Autodesk Inventor part; units mm, degrees
ref_plane "YZ Plane" through (0, 0, 0) normal (1, 0, 0) x (0, 1, 0)
ref_plane "XZ Plane" through (0, 0, 0) normal (0, 1, 0) x (-1, 0, 0)
ref_plane "XY Plane" through (0, 0, 0) normal (0, 0, 1) x (1, 0, 0)
sketch "Sketch1" plane through (0, 0, 0) normal (0, 1, 0) x (-1, 0, 0)
  line L0 (63.6448, -68.929) -> (37.6448, -68.929)
  line L1 (37.6448, -68.929) -> (37.6448, -42.929)
  line L2 (37.6448, -42.929) -> (63.6448, -42.929)
  line L3 (63.6448, -42.929) -> (63.6448, -68.929)
  point P0 (0, 0)
  dimension "d0" = 26
  dimension "d1" = 26
extrude "Extrusion1" add sketch "Sketch1" along normal blind 1.2
sketch "Sketch2" plane through (0, 1.2, 0) normal (0, 1, 0) x (1, 0, 0)
  line L0 (-63.6448, 68.929) -> (-63.6448, 42.929)
  line L1 (-37.6448, 42.929) -> (-37.6448, 68.929)
  line L2 (-63.6448, 64.229) -> (-37.6448, 64.229)
  line L3 (-37.6448, 64.229) -> (-37.6448, 47.629)
  line L4 (-37.6448, 47.629) -> (-63.6448, 47.629)
  line L5 (-63.6448, 47.629) -> (-63.6448, 64.229)
  line L6 (-37.6448, 68.929) -> (-63.6448, 68.929)
  point P0 (0, 0)
  point P1 (-63.6448, 47.629)
  dimension "d4" = 4.7
  dimension "d5" = 16.6
extrude "Extrusion2" add sketch "Sketch2" along normal blind 2 contours L2 L1 L4 L0
sketch "Sketch3" plane through (0, 1.2, 0) normal (0, 1, 0) x (1, 0, 0)
  circle A0 centre (-61.6448, 66.929) radius 1
  circle A1 centre (-39.6448, 66.929) radius 1
  circle A2 centre (-39.6448, 44.929) radius 1
  circle A3 centre (-61.8448, 44.929) radius 1
  line L0 (-63.6448, 68.929) -> (-63.6448, 64.229)
  line L1 (-37.6448, 68.929) -> (-63.6448, 68.929)
  line L2 (-37.6448, 64.229) -> (-37.6448, 68.929)
  line L3 (-37.6448, 42.929) -> (-37.6448, 47.629)
  line L4 (-63.6448, 42.929) -> (-37.6448, 42.929)
  line L5 (-63.6448, 47.629) -> (-63.6448, 42.929)
  point P0 (0, 0)
  point P1 (-63.6448, 45.279)
  dimension "d8" = 2
  dimension "d9" = 2
  dimension "d10" = 2
  dimension "d11" = 2
  dimension "d12" = 2
  dimension "d13" = 2
  dimension "d14" = 2
  dimension "d15" = 2
  dimension "d16" = 2
  dimension "d17" = 2
  dimension "d18" = 2
  dimension "d19" = 1.8
extrude "Extrusion3" cut sketch "Sketch3" against normal through all
sketch "Sketch4" plane through (0, 0, 0) normal (0, -1, 0) x (1, 0, 0)
  line L0 (-45.8948, -68.929) -> (-55.8948, -68.929)
  line L1 (-55.8948, -68.929) -> (-55.8948, -66.429)
  line L2 (-55.8948, -66.429) -> (-45.8948, -66.429)
  line L3 (-45.8948, -66.429) -> (-45.8948, -68.929)
  line L4 (-37.6448, -68.929) -> (-63.6448, -68.929)
  line L5 (-37.6448, -42.929) -> (-37.6448, -68.929)
  point P0 (0, 0)
  dimension "d22" = 10
  dimension "d23" = 2.5
  dimension "d24" = 0
  dimension "d25" = 8.25
extrude "Extrusion4" add sketch "Sketch4" along normal blind 2.5
sketch "Sketch5" plane through (0, -2.5, 0) normal (0, -1, 0) x (1, 0, 0)
  line L0 (-64.9448, -68.229) -> (-76.9448, -68.229)
  line L1 (-76.9448, -68.229) -> (-76.9448, -56.229)
  line L2 (-76.9448, -56.229) -> (-64.9448, -56.229)
  line L3 (-64.9448, -56.229) -> (-64.9448, -68.229)
  line L4 (-64.9448, -55.629) -> (-76.9448, -55.629)
  line L5 (-76.9448, -55.629) -> (-76.9448, -43.629)
  line L6 (-76.9448, -43.629) -> (-64.9448, -43.629)
  line L7 (-64.9448, -43.629) -> (-64.9448, -55.629)
  line L8 (-55.8948, -68.929) -> (-63.6448, -68.929)
  line L9 (-63.6448, -68.929) -> (-63.6448, -42.929)
  line L10 (-63.6448, -42.929) -> (-37.6448, -42.929)
  point P0 (0, 0)
  dimension "d28" = 12
  dimension "d29" = 12
  dimension "d30" = 12
  dimension "d31" = 12
  dimension "d32" = 0.7
  dimension "d33" = 1.3
  dimension "d34" = 0.7
extrude "Extrusion5" add sketch "Sketch5" against normal blind 3.7
sketch "Sketch7" plane through (0, 1.2, 0) normal (0, 1, 0) x (1, 0, 0)
  circle A0 centre (-70.9448, 62.229) radius 3.25
  circle A1 centre (-70.9448, 49.629) radius 3.25
  line L0 (-64.9448, 68.229) -> (-76.9448, 68.229)
  line L1 (-76.9448, 68.229) -> (-76.9448, 43.629)
  line L2 (-64.9448, 55.629) -> (-76.9448, 55.629)
  line L3 (-76.9448, 55.629) -> (-76.9448, 43.629)
  point P0 (0, 0)
  point P1 (-76.9448, 56.229)
  dimension "d47" = 6.5
  dimension "d48" = 6.5
  dimension "d49" = 6
  dimension "d50" = 6
  dimension "d51" = 6
  dimension "d52" = 6
extrude "Extrusion7" add sketch "Sketch7" along normal blind 8.8
draft "FaceDraft3" angle 2.5 pull direction (0, 1, 0) faces at (-67.7053, 7.0667, -61.9675) fixed edges at (-74.1948, 1.2, -62.229)
draft "FaceDraft4" angle 2.5 pull direction (0, 1, 0) faces at (-67.7053, 7.0667, -49.3675) fixed edges at (-74.1948, 1.2, -49.629)
sketch "Sketch8" plane through (0, -2.5, 0) normal (0, -1, 0) x (1, 0, 0)
  line L0 (-78.2948, -34.929) -> (-36.2948, -34.929)
  line L1 (-36.2948, -34.929) -> (-36.2948, -76.929)
  line L2 (-36.2948, -76.929) -> (-78.2948, -76.929)
  line L3 (-78.2948, -76.929) -> (-78.2948, -34.929)
  line L4 (-63.6448, -42.929) -> (-37.6448, -42.929)
  line L5 (-37.6448, -42.929) -> (-37.6448, -68.929)
  circle A0 centre (-74.7948, -73.429) radius 1.75
  circle A1 centre (-39.7948, -73.429) radius 1.75
  circle A2 centre (-74.7948, -38.429) radius 1.75
  circle A3 centre (-39.7948, -38.429) radius 1.75
  line L6 (-37.6448, -47.629) -> (-37.6448, -64.229)
  point P0 (0, 0)
  point P1 (-37.6448, -55.929)
  dimension "d57" = 42
  dimension "d58" = 42
  dimension "d59" = 8
  dimension "d63" = 3.5
  dimension "d64" = 3.5
  dimension "d65" = 3.5
  dimension "d66" = 3.5
  dimension "d67" = 3.5
  dimension "d68" = 3.5
  dimension "d69" = 3.5
  dimension "d70" = 3.5
  dimension "d71" = 3.5
  dimension "d72" = 3.5
  dimension "d73" = 3.5
  dimension "d74" = 3.5
  dimension "d75" = 1.35
extrude "Extrusion8" add sketch "Sketch8" along normal blind 1.6
equation "\"d14\" = d13"
equation "\"d15\" = d14"
equation "\"d16\" = d14"
equation "\"d17\" = d15"
equation "\"d18\" = d12"
equation "\"d51\" = d49"
equation "\"d52\" = d50"
equation "\"d64\" = d63"
equation "\"d65\" = d63"
equation "\"d66\" = d63"
equation "\"d68\" = d67"
equation "\"d69\" = d68"
equation "\"d70\" = d68"
equation "\"d71\" = d69"
equation "\"d72\" = d70"
equation "\"d73\" = d67"
equation "\"d74\" = d68"
properties part number "display_buttons"
The model under review builds one solid part; all positions refer to its coordinate system, in mm. A direction names the side the tool comes from. Coordinates: 2 decimals unless noted, no trailing zeros. Write each loop counter-clockwise with the first axis right and the second up, starting at its lowest first coordinate (ties: lowest second). Pieces come first, ordered by that corner, then holes.
1) Machinability: for faces 4 (the face through (-51, 0, -68.929)), 5 (the face through (-64.945, -1, -62)), 6 (the face through (-74, 1.2, -52)), 7 (the face through (-50, 2, -47.629)), which of the approach directions +Z, -Z, +X, -X, +Y, -Y give a long, thin tool a straight path to every point of the face, cutting with its end or side? Answer none if there is none.
2) To check wall thickness, follow probe 1 along Z at (x, y) = (-71.5, 9); probe 2 along Z at (x, y) = (-71.5, -2.25); probe 3 along Y at (x, z) = (-60.5, -64.5). State the ranges of each line that lie inside material, in increasing order.
3) We need section D-D on y = 7.5. State the section outline as (x, z) points.
4) We need section B-B on x = -47. State the section outline as (y, z) points.
5) We need section A-A on y = -1.25. State the section outline as (x, z) points, then the cut area to 3 significant figures.
6) The part is to be moulded in two halves that separate along X. For faces 1 (the face through (-39.183, 0.608, -44.042)), 2 (the face through (-71, -1, -43.629)), 3 (the face through (-78.295, -3, -56)), say which applies: pulls with the +X half, pulls with the -X half, needs draft (parallel to the pull), parting line crosses it, or undercut.
7) We need section C-C on z = -37.5. State the section outline as (x, y) points, then the cut area to 3 significant figures.
8) Clearance check with flat-ended pins moving along their axes: pin 1 Ø6 at (y, z) = (3.5, -61.5) entering from -X; pin 2 Ø1 at (y, z) = (1.5, -59.5) entering from +X; pin 3 Ø5 at (x, z) = (-46.5, -45.5) entering from +Y. State where each tip first meets the part, or that it passes through.
Answer list:
1. face 4: -Z, +X, -X, +Y
1. face 5: +Z, -Z, +Y
1. face 6: +Y
1. face 7: +Z, +X, +Y
2. probe 1: z = -65.08 to -59.37, -52.48 to -46.77
2. probe 2: z = -68.23 to -56.23, -55.63 to -43.63
2. probe 3: y = -4.1 to -2.5, 0 to 1.2
3. outline: circle Ø5.95 at (-70.94, -62.23); circle Ø5.95 at (-70.94, -49.63)
4. outline: (-4.1, -76.93) - (-2.5, -76.93) - (-2.5, -68.93) - (1.2, -68.93) - (1.2, -64.23) - (3.2, -64.23) - (3.2, -47.63) - (1.2, -47.63) - (1.2, -42.93) - (0, -42.93) - (0, -66.43) - (-2.5, -66.43) - (-2.5, -34.93) - (-4.1, -34.93) - close
5. outline: (-76.94, -68.23) - (-64.94, -68.23) - (-64.94, -56.23) - (-76.94, -56.23) - close; (-76.94, -55.63) - (-64.94, -55.63) - (-64.94, -43.63) - (-76.94, -43.63) - close; (-55.89, -68.93) - (-45.89, -68.93) - (-45.89, -66.43) - (-55.89, -66.43) - close
5. area: 313 mm2
6. face 1: undercut
6. face 2: needs draft
6. face 3: pulls with the -X half
7. outline: (-78.29, -4.1) - (-76.28, -4.1) - (-76.28, -2.5) - (-78.29, -2.5) - close; (-73.31, -4.1) - (-41.28, -4.1) - (-41.28, -2.5) - (-73.31, -2.5) - close; (-38.31, -4.1) - (-36.29, -4.1) - (-36.29, -2.5) - (-38.31, -2.5) - close
7. area: 57.7 mm2
8. pin 1: stops at x = -76.94
8. pin 2: stops at x = -37.64
8. pin 3: stops at y = 3.2
